The listing builds one solid part. Answer for the finished solid, in the listing's coordinates (mm). Give positions to 0.01 mm unless a question says otherwise; leave off trailing zeros. Write each loop counter-clockwise with the first axis right and the second up, starting at its lowest first coordinate (ties: lowest second). Pieces come first, ordered by that corner, then holes. Notation, with made-up numbers: (-11.5, -29) - (-3.5, -29) arc R23 ccw to (-3.5, 4) - close; hole circle Ø6 at (-12, 64). An arc over 180 degrees is marked (long way). One line per question, with ' | ' between items. Start each with the question number.
1. A cutting plane is placed at C-C (x = 3). Determine the outline of the cut face in (y, z) (3 decimals).
2. A cutting plane is placed at A-A (x = 38.5). Determine the outline of the cut face in (y, z) (3 decimals), then the cut area to 3 significant figures.
3. Find the intervals of material crossed by L1, parallel to Z at x = 61, y = 1.85; L2, parallel to Z at x = -50.5, y = 2.25; L3, parallel to X at y = 2.7, z = 29.5, in increasing order. Write a range as from..to.
4. Given P1, Ø4, axis at x = -52, z = 27.5, coming from the -Y side; P2, Ø1.6, axis at x = -62, y = 2, coming from the +Z side; P3, Ø1.6, axis at x = 37, y = 1, coming from the -Z side; P4, Ø6, axis at x = 17.49, z = 3.49, coming from the +Y side, each flat-ended and moving along its own axis, determine where each tip first touches the part or whether it passes through.
5. A cutting plane is placed at B-B (z = -41). Determine the outline of the cut face in (x, y) (3 decimals), then the cut area to 3 significant figures.
6. A cutting plane is placed at D-D (y = 0.75). State how many separate pieces and enclosed holes the cut face has, then the cut area to 4 significant figures.
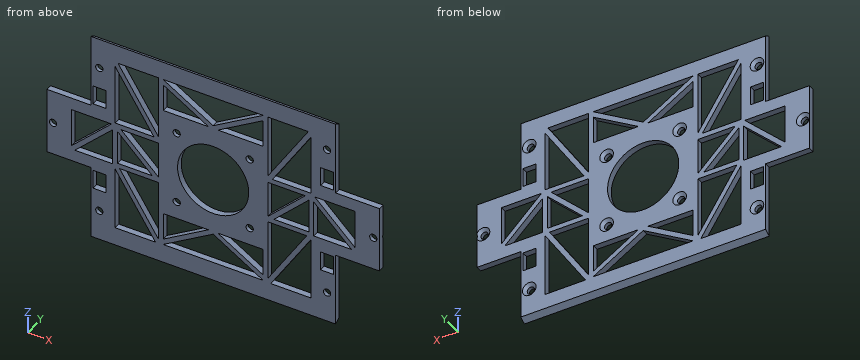
```python
from build123d import *

# Parameters (mm, degrees)
SKETCH1_R                                         = 18.5801
BOSS_EXTRUDE1_DEPTH                               = 3.175
CSK_FOR_6_FLAT_HEAD_MACHINE_SCREW_100_D           = 3.7973
CSK_FOR_6_FLAT_HEAD_MACHINE_SCREW_100_CSINK_D     = 7.0866
CSK_FOR_6_FLAT_HEAD_MACHINE_SCREW_100_CSINK_ANGLE = 100
CUT_EXTRUDE2_DEPTH                                = 114.138623562
SKETCH7_W                                         = 6.7056
SKETCH7_H                                         = 9.8806
CUT_EXTRUDE5_DEPTH                                = 114.138623562


with BuildPart() as part:
    # Sketch1 → Boss-Extrude1 (new body)
    with BuildSketch(Plane(origin=(0, 0, 0), x_dir=(1, 0, 0), z_dir=(0, 1, 0))):
        Polygon((-65.455327335, 70.644677608), (62.306672665, 70.644677608), (62.306672665, 32.544677608), (85.166672665, 32.544677608), (85.166672665, -1.999322392), (62.306672665, -1.999322392), (62.306672665, -40.099322392), (-65.455327335, -40.099322392), (-65.455327335, -1.999322392), (-88.315327335, -1.999322392), (-88.315327335, 32.544677608), (-65.455327335, 32.544677608), align=None)
        with Locations(Location((-1.574327335, 15.145677608, 0), (0, 0, 270))):
            Circle(SKETCH1_R, mode=Mode.SUBTRACT)
    extrude(amount=BOSS_EXTRUDE1_DEPTH)

    # CSK for #6 Flat Head Machine Screw (100)1 (through all)
    with Locations(Plane(origin=(0, 3.175, 0), x_dir=(1, 0, 0), z_dir=(0, 1, 0))):
        with Locations((-60.978577335, 54.896669208), (-85.108577335, 15.336169208), (-60.978577335, -24.224330792), (57.861672665, -24.224322392), (81.991672665, 15.336177608), (57.861672665, 54.896677608), (-20.608452335, 34.608427608), (-20.608452335, -3.491572392), (17.491547665, -3.491572392), (17.491547665, 34.608427608)):
            CounterSinkHole(CSK_FOR_6_FLAT_HEAD_MACHINE_SCREW_100_D / 2, CSK_FOR_6_FLAT_HEAD_MACHINE_SCREW_100_CSINK_D / 2, counter_sink_angle=CSK_FOR_6_FLAT_HEAD_MACHINE_SCREW_100_CSINK_ANGLE)

    # Sketch4 → Cut-Extrude2 (cut, symmetric)
    with BuildSketch(Plane(origin=(0, 0, 0), x_dir=(0, 0, -1), z_dir=(1, 0, 0))):
        Polygon((70.644677608, 0), (68.811590503, 3.175), (70.644677608, 3.175), align=None)
    cut_extrude2 = extrude(amount=CUT_EXTRUDE2_DEPTH, both=True, mode=Mode.SUBTRACT)

    # Mirror1: Cut-Extrude2 across plane
    add(cut_extrude2.mirror(Plane.XY.offset(-15.272677608)), mode=Mode.SUBTRACT)

    # Sketch7 → Cut-Extrude5 (cut, through all)
    with BuildSketch(Plane(origin=(0, 3.175, 0), x_dir=(1, 0, 0), z_dir=(0, 1, 0))):
        Polygon((-31.662153757, 61.119677608), (-52.755327335, 61.119677608), (-52.755327335, 28.53190944), align=None)
        Polygon((-30.149327335, 58.782445776), (-50.420464549, 27.464677608), (-30.149327335, 27.464677608), align=None)
        Polygon((-54.025327335, 7.320825628), (-54.025327335, 26.194677608), (-73.777032895, 26.194677608), align=None)
        Polygon((-27.609327335, 60.865677608), (-27.609327335, 60.822739389), (-1.574327335, 45.201739389), (-1.574327335, 60.865677608), align=None)
        Polygon((-30.149327335, 5.620677608), (-30.149327335, 24.428637467), (-49.613378817, 5.620677608), align=None)
        Polygon((-33.291275852, 24.924677608), (-51.485327335, 24.924677608), (-51.485327335, 7.34390876), align=None)
        Polygon((-27.609327335, 57.860615827), (-27.609327335, 43.720677608), (-4.042763637, 43.720677608), align=None)
        Polygon((-54.593621774, 4.350677608), (-75.615327335, 24.438085143), (-75.615327335, 4.350677608), align=None)
        Polygon((-32.48419012, 3.080677608), (-52.755327335, 3.080677608), (-52.755327335, -28.23709056), align=None)
        Polygon((-30.149327335, -30.574322392), (-30.149327335, 2.013445776), (-51.242500913, -30.574322392), align=None)
        Polygon((-4.042763637, -13.429322392), (-27.609327335, -13.429322392), (-27.609327335, -27.569260611), align=None)
        Polygon((-27.609327335, -30.531384173), (-27.609327335, -30.574322392), (-1.574327335, -30.574322392), (-1.574327335, -14.910384173), align=None)
        with Locations((-60.978577335, -8.099133955)):
            Rectangle(SKETCH7_W, SKETCH7_H)
        with Locations((-60.978577335, 38.644472371)):
            Rectangle(SKETCH7_W, SKETCH7_H)
    cut_extrude5 = extrude(amount=-CUT_EXTRUDE5_DEPTH, mode=Mode.SUBTRACT)

    # Mirror3: Cut-Extrude5 across plane
    add(cut_extrude5.mirror(Plane(origin=(-1.574327335, 0, 0), x_dir=(0, 0, 1), z_dir=(1, 0, 0))), mode=Mode.SUBTRACT)


solid = part.part
```
Determined:
1) outline: (0, -70.645) - (3.175, -68.812) - (3.175, -60.866) - (0, -60.866) - close; (0, -47.946) - (3.175, -47.946) - (3.175, -44.984) - (0, -44.984) - close; (0, -43.721) - (3.175, -43.721) - (3.175, -33.154) - (0, -33.154) - close; (0, 2.863) - (3.175, 2.863) - (3.175, 13.429) - (0, 13.429) - close; (0, 14.693) - (3.175, 14.693) - (3.175, 17.655) - (0, 17.655) - close; (0, 30.574) - (3.175, 30.574) - (3.175, 38.266) - (0, 40.099) - close
2) outline: (0, -70.645) - (3.175, -68.812) - (3.175, -61.12) - (0, -61.12) - close; (0, -45.691) - (3.175, -45.691) - (3.175, -41.017) - (0, -41.017) - close; (0, -27.465) - (3.175, -27.465) - (3.175, -24.925) - (0, -24.925) - close; (0, -16.849) - (3.175, -16.849) - (3.175, -13.317) - (0, -13.317) - close; (0, -5.621) - (3.175, -5.621) - (3.175, -3.081) - (0, -3.081) - close; (0, 11.078) - (3.175, 11.078) - (3.175, 15.752) - (0, 15.752) - close; (0, 30.574) - (3.175, 30.574) - (3.175, 38.266) - (0, 40.099) - close | area: 112 mm2
3) L1: -69.58..-43.58, -33.7..-26.19, -16.99..-13.48, -4.35..3.16, 13.04..39.03 | L2: -69.35..-61.12, -32.02..-24.92, -8.3..-3.08, 24.75..29.43, 30.57..38.8 | L3: -65.46..-50.55, -30.15..-25.89, 22.74..27, 47.4..62.31
4) P1: y = 0 | P2: z = 39.41 | P3: z = -70.53 | P4: y = 2.72
5) outline: (-65.455, 0) - (-64.331, 0) - (-64.331, 3.175) - (-65.455, 3.175) - close; (-57.626, 0) - (-52.755, 0) - (-52.755, 3.175) - (-57.626, 3.175) - close; (-44.685, 0) - (-41.659, 0) - (-41.659, 3.175) - (-44.685, 3.175) - close; (-30.149, 0) - (27.001, 0) - (27.001, 3.175) - (-30.149, 3.175) - close; (38.511, 0) - (41.536, 0) - (41.536, 3.175) - (38.511, 3.175) - close; (49.607, 0) - (54.477, 0) - (54.477, 3.175) - (49.607, 3.175) - close; (61.183, 0) - (62.307, 0) - (62.307, 3.175) - (61.183, 3.175) - close | area: 239 mm2
6) separate pieces: 1 | enclosed holes: 37 | area: 8,545 mm2
